```python
from build123d import *

# Parameters (mm, degrees)
SKETCH1_W          = 63.5
SKETCH1_H          = 57.15
SKETCH1_R          = 19.8628
EXTRUDE1_DEPTH     = 44.45
CUT_EXTRUDE1_DEPTH = 64.5
SKETCH3_R          = 22.225
CUT_EXTRUDE2_DEPTH = 31.75
FILLET1_R          = 1.524
HOLE1_D            = 7.1374
HOLE1_DEPTH        = 57.15


with BuildPart() as part:
    # Sketch1 → Extrude1 (new body)
    with BuildSketch(Plane.XY):
        with Locations((0, 28.575)):
            Rectangle(SKETCH1_W, SKETCH1_H)
        with Locations((0, 28.575)):
            Circle(SKETCH1_R, mode=Mode.SUBTRACT)
    extrude(amount=-EXTRUDE1_DEPTH)

    # Sketch2 → Cut-Extrude1 (cut, through all)
    with BuildSketch(Plane(origin=(31.75, 0, 0), x_dir=(0, 0, -1), z_dir=(1, 0, 0))):
        Polygon((12.7, 57.15), (44.45, 2.286), (44.45, 57.15), align=None)
    extrude(amount=-CUT_EXTRUDE1_DEPTH, mode=Mode.SUBTRACT)

    # Sketch3 → Cut-Extrude2 (cut)
    with BuildSketch(Plane(origin=(0, 0, -44.45), x_dir=(-1, 0, 0), z_dir=(0, 0, -1))):
        with Locations(Location((0, 28.575, 0), (0, 0, 270))):  # turned: the seam where the file's is
            Circle(SKETCH3_R)
    extrude(amount=-CUT_EXTRUDE2_DEPTH, mode=Mode.SUBTRACT)

    # Fillet1
    fillet1_edges = [part.edges().sort_by_distance(p)[0] for p in [
        (0, 50.8, -12.7),
    ]]
    fillet(fillet1_edges, radius=FILLET1_R)

    # Hole1
    with Locations(Plane(origin=(0, 57.15, 0), x_dir=(-1, 0, 0), z_dir=(0, 1, 0))):
        with Locations((25.4, -6.35), (-25.4, -6.35)):
            Hole(HOLE1_D / 2, depth=HOLE1_DEPTH)


solid = part.part
```
Check sheet for the modelled part. Datum: model origin and axes. Units: mm. A direction names the side the tool comes from. Coordinates: 2 decimals unless noted, no trailing zeros. Write each loop counter-clockwise with the first axis right and the second up, starting at its lowest first coordinate (ties: lowest second). Pieces come first, ordered by that corner, then holes. Notation, with made-up numbers: M 4,-12.5 L 25,-12.5 A13 cw 25,2.5 Z; hole C -32,59.5 d8. An arc over 180 degrees is marked long. Write item = value, one per line. Start each with the question number.
1. Tool access check on faces 5 (the cylindrical face through (-6.676, 7.376, -25.259)), 6 (the flat face through (-8, 48, 0)). Record the directions out of +Z, -Z, +X, -X, +Y, -Y that give a thin tool (end or side, any length) a straight path to the whole face; none if there is none.
2. Thickness scan on probe 1 along X at (y, z) = (38, -5.5); probe 2 along X at (y, z) = (20, -6); probe 3 along Z at (x, y) = (-27.5, 10.5). Record the ranges inside material, lowest first.
3. Sectioned sample at C-C (y = 24). State how many separate pieces and enclosed holes the cut face has, then the cut area to 3 significant figures.
4. Sectioned sample at D-D (x = 0). Record the cut outline in (y, z), then the cut area to 3 significant figures.
5. Sectioned sample at A-A (x = -25.4). Record the cut outline in (y, z), then the cut area to 3 significant figures.
6. Sectioned sample at B-B (z = -6.35). Record the cut outline in (x, y) (3 decimals), then the cut area to 3 significant figures.
7. Go/stop test with a flat-tipped pin: pin 1 (6.5 mm diameter, centred on x = 25.4, z = -6.35, fed in from +Y). Record where the tip stops, or that it passes through.
8. Mould release check, pull along Y, two halves, no side actions. Record for faces 1 (the flat face through (-18.5, 36.3, -12.7)), 2 (the flat face through (0, 0, -22)), 3 (the flat face through (21.611, 36.198, -24.825)), 4 (the flat face through (0, 1, -44.45)): pulls with the +Y half, pulls with the -Y half, needs draft (parallel to the pull), parting line crosses it, or undercut.
The answers:
q1.face_5 = -Z
q1.face_6 = +Z, +X, -X, +Y, -Y
q2.probe_1 = -31.75 to -28.87, -21.93 to -17.48, 17.48 to 21.93, 28.87 to 31.75
q2.probe_2 = -31.75 to -28.95, -21.85 to -17.92, 17.92 to 21.85, 28.95 to 31.75
q2.probe_3 = -39.7 to -9.24, -3.46 to 0
q3.separate_pieces = 2
q3.enclosed_holes = 2
q3.area = 620 mm²
q4.outline = M 0,-44.45 L 2.29,-44.45 L 6.35,-42.1 L 6.35,-14.22 A1.52 cw 7.87,-12.7 L 8.71,-12.7 L 8.71,0 L 0,0 Z; M 48.44,-12.7 L 49.28,-12.7 A1.52 cw 50.8,-14.22 L 50.8,-16.37 L 57.15,-12.7 L 57.15,0 L 48.44,0 Z
q4.area = 431 mm²
q5.outline = M 0,-44.45 L 2.29,-44.45 L 57.15,-12.7 L 57.15,-9.92 L 0,-9.92 Z; M 0,-2.78 L 57.15,-2.78 L 57.15,0 L 0,0 Z
q5.area = 1,260 mm²
q6.outline = M -31.75,0 L -28.969,0 L -28.969,57.15 L -31.75,57.15 Z; M -21.831,0 L 21.831,0 L 21.831,57.15 L -21.831,57.15 Z; M 28.969,0 L 31.75,0 L 31.75,57.15 L 28.969,57.15 Z; hole C 0,28.575 d39.726
q6.area = 1,570 mm²
q7.pin_1 = through
q8.face_1 = undercut
q8.face_2 = pulls with the -Y half
q8.face_3 = pulls with the +Y half
q8.face_4 = needs draft
